Verification items for the finished model (mm, model axes). Face numbers are marked on the shaded views. A direction names the side the tool comes from. Give positions to 0.01 mm unless a question says otherwise; leave off trailing zeros. Write each loop counter-clockwise with the first axis right and the second up, starting at its lowest first coordinate (ties: lowest second). Pieces come first, ordered by that corner, then holes. Notation, with made-up numbers: (-38.75, -38) -> (-23.75, -38) arc R22 cw to (-23.75, 1) -> close; hole circle Ø1 at (55.25, 0). An arc over 180 degrees is marked (long way). Answer as CSV lines item,"result". Start each with the question number.
1) Tool access check on the marked faces 1, 2 and 3. Record the directions out of +Z, -Z, +X, -X, +Y, -Y that give a thin tool (end or side, any length) a straight path to the whole face; none if there is none.
2) Gauge pin test, flat ends, axial feed: pin 1 Ø6 at (y, z) = (17.5, 1) entering from -X; pin 2 Ø6.5 at (x, z) = (41.5, -2) entering from -Y; pin 3 Ø5 at (x, z) = (0, 0) entering from +Y. Record the tip position at first contact, or that the pin passes through.
3) Material ranges on L1, parallel to X at y = 18, z = 0.5; L2, parallel to Z at x = 0, y = 37.1; L3, parallel to X at y = 17, z = 0.5, recorded low to high.
4) Sectioned sample at B-B on x = 16. Record the cut outline in (y, z).
5) Sectioned sample at C-C on x = 0. Record the cut outline in (y, z), and give its area (3 significant figures).
6) Mould release check, pull along Z, two halves, no side actions. Record for the marked faces 4, 5 and 6: released by +Z, released by -Z, zero draft, split by the parting line, or undercut.
7) Sectioned sample at A-A on y = 24.5. Record the cut outline in (x, z), and give its area (3 significant figures).
8) Sectioned sample at D-D on x = 39.5. Record the cut outline in (y, z).
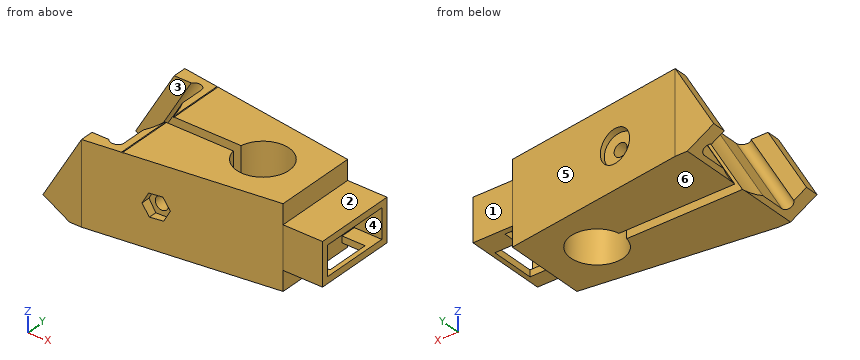
```python
from build123d import *

# Parameters (mm, degrees)
BOSS_EXTRUDE1_DEPTH     = 40
CUT_EXTRUDE1_DEPTH      = 40
SKETCH3_W               = 4.376715803
SKETCH3_H               = 7.921330006
BOSS_EXTRUDE2_DEPTH     = 40
CUT_EXTRUDE2_DEPTH      = 78.145313728
CUT_EXTRUDE2_DEPTH_BACK = 78.145313728
CUT_EXTRUDE3_DEPTH      = 40
CUT_EXTRUDE4_DEPTH      = 43.935998882
CUT_EXTRUDE4_DEPTH_BACK = 43.935998882
SKETCH6_R               = 2
CUT_EXTRUDE5_DEPTH      = 5
SKETCH8_R               = 5
CUT_EXTRUDE6_DEPTH      = 5
CUT_EXTRUDE7_START      = -2
SKETCH9_W               = 6.222682415
SKETCH9_H               = 53.403341902
CUT_EXTRUDE7_DEPTH      = 16
SKETCH10_W              = 13
SKETCH10_H              = 25
SKETCH10_W_2            = 9
SKETCH10_H_2            = 21
BOSS_EXTRUDE3_DEPTH     = 12
CUT_EXTRUDE8_DEPTH      = 11


with BuildPart() as part:
    # Sketch1 → Boss-Extrude1 (new body)
    with BuildSketch(Plane(origin=(0, 0, 0), x_dir=(1, 0, 0), z_dir=(0, 1, 0))):
        Polygon((-35, 12.5), (-20.56624327, -12.5), (35, -12.5), (35, 12.5), align=None)
    extrude(amount=BOSS_EXTRUDE1_DEPTH)

    # Sketch2 → Cut-Extrude1 (cut)
    with BuildSketch(Plane.XY.offset(12.5)):
        Polygon((-20.56624327, 40), (35, 32.5), (35, 40), align=None)
        Polygon((35, 7.5), (-20.56624327, 0), (35, 0), align=None)
    extrude(amount=-CUT_EXTRUDE1_DEPTH, mode=Mode.SUBTRACT)

    # Sketch3 → Boss-Extrude2 (add)
    with BuildSketch(Plane(origin=(-20.837341226, 0, 12.030444566), x_dir=(0.4999999999999981, 0, 0.8660254037844397), z_dir=(-0.8660254037844398, 0, 0.4999999999999982))):
        with Locations((-10.675795445, 21.421253709)):
            Rectangle(SKETCH3_W, SKETCH3_H)
    extrude(amount=BOSS_EXTRUDE2_DEPTH)

    # Sketch4 → Cut-Extrude2 (cut, two sides: drawn at the far end of the back side and taken through both)
    with BuildSketch(Plane(origin=(-4.243718771, 0, -7.350336525), x_dir=(0.8660254037844397, 0, -0.4999999999999983), z_dir=(0.4999999999999982, 0, 0.8660254037844396)).offset(-CUT_EXTRUDE2_DEPTH_BACK)):
        with BuildLine():
            Line((-25.260889132, 35.934120187), (-19.597573928, 35.934120187))
            ThreePointArc((-19.597573928, 35.934120187), (-17.574079433, 36.729704946), (-16.260889132, 34.996783621))
            Line((-16.260889132, 34.996783621), (-16.260889132, 27.623217913))
            ThreePointArc((-16.260889132, 27.623217913), (-14.610889132, 19.996783621), (-16.260889132, 12.37034933))
            Line((-16.260889132, 12.37034933), (-16.260889132, 4.996783621))
            ThreePointArc((-16.260889132, 4.996783621), (-17.574079433, 3.263862297), (-19.597573928, 4.059447055))
            Line((-19.597573928, 4.059447055), (-25.260889132, 4.059447055))
            Line((-25.260889132, 4.059447055), (-25.260889132, 11.549622397))
            Line((-25.260889132, 11.549622397), (-69.354192402, 11.549622397))
            Line((-69.354192402, 11.549622397), (-69.354192402, 27.546843348))
            Line((-69.354192402, 27.546843348), (-25.260889132, 26.613076168))
            Line((-25.260889132, 26.613076168), (-25.260889132, 35.934120187))
        make_face()
    extrude(amount=CUT_EXTRUDE2_DEPTH + CUT_EXTRUDE2_DEPTH_BACK, mode=Mode.SUBTRACT)

    # Sketch5 → Cut-Extrude3 (cut)
    with BuildSketch(Plane(origin=(0, 0, -12.5), x_dir=(-1, 0, 0), z_dir=(0, 0, -1))):
        with BuildLine():
            Line((-11.141275202, 21.5), (29.874932975, 21.5))
            Line((29.874932975, 21.5), (29.874932975, 18.5))
            Line((29.874932975, 18.5), (-11.142492493, 18.5))
            ThreePointArc((-11.142492493, 18.5), (-26.999999341, 20.006434648), (-11.141275202, 21.5))
        make_face()
    extrude(amount=-CUT_EXTRUDE3_DEPTH, mode=Mode.SUBTRACT)

    # Sketch6 → Cut-Extrude4 (cut, two sides: drawn at the far end of the back side and taken through both)
    with BuildSketch(Plane(origin=(0, 18.5, 0), x_dir=(1, 0, 0), z_dir=(0, 1, 0)).offset(-CUT_EXTRUDE4_DEPTH_BACK)):
        Circle(SKETCH6_R)
    extrude(amount=CUT_EXTRUDE4_DEPTH + CUT_EXTRUDE4_DEPTH_BACK, mode=Mode.SUBTRACT)

    # Sketch7 → Cut-Extrude5 (cut)
    with BuildSketch(Plane.XZ):
        Polygon((1.8525736, 3.461402084), (-2.071375338, 3.335076842), (-3.923948938, -0.126325242), (-1.8525736, -3.461402084), (2.071375338, -3.335076842), (3.923948938, 0.126325242), align=None)
    extrude(amount=-CUT_EXTRUDE5_DEPTH, mode=Mode.SUBTRACT)

    # Sketch8 → Cut-Extrude6 (cut)
    with BuildSketch(Plane(origin=(0, 40, 0), x_dir=(1, 0, 0), z_dir=(0, 1, 0))):
        with Locations(Location((0, 0, 0), (0, 0, 270))):
            Circle(SKETCH8_R)
    extrude(amount=-CUT_EXTRUDE6_DEPTH, mode=Mode.SUBTRACT)

    # Sketch9 → Cut-Extrude7 (cut)
    with BuildSketch(Plane(origin=(-14.082343077, 0, 8.130444566), x_dir=(0.4999999999999982, 0, 0.8660254037844397), z_dir=(-0.8660254037844398, 0, 0.4999999999999983)).offset(CUT_EXTRUDE7_START)):
        with Locations((-26.065813196, 19.047949313)):
            Rectangle(SKETCH9_W, SKETCH9_H)
        Polygon((6.045528012, 45.749620264), (6.045528012, -7.653721638), (13.717164193, -7.653721638), (13.717164193, 42.686575292), (13.717164193, 45.749620264), align=None)
    extrude(amount=CUT_EXTRUDE7_DEPTH, mode=Mode.SUBTRACT)

    # Sketch10 → Boss-Extrude3 (add)
    with BuildSketch(Plane(origin=(35, 0, 0), x_dir=(0, 0, -1), z_dir=(1, 0, 0))):
        with Locations((0, 20)):
            Rectangle(SKETCH10_W, SKETCH10_H)
        with Locations((0, 20)):
            Rectangle(SKETCH10_W_2, SKETCH10_H_2, mode=Mode.SUBTRACT)
    extrude(amount=BOSS_EXTRUDE3_DEPTH)

    # Sketch11 → Cut-Extrude8 (cut)
    with BuildSketch(Plane(origin=(0, 0, -6.5), x_dir=(-1, 0, 0), z_dir=(0, 0, -1))):
        Polygon((-38.6, 30.8), (-35, 30.8), (-35, 25.8), (-35, 12.2), (-35, 9.2), (-38.6, 9.2), (-38.6, 12.2), (-45.6, 12.2), (-45.6, 25.8), (-38.6, 25.8), align=None)
    extrude(amount=-CUT_EXTRUDE8_DEPTH, mode=Mode.SUBTRACT)


solid = part.part
```
Ans:
1,face 1,"+Z, -Z, +X, +Y"
1,face 2,"+Z, +X, +Y, -Y"
1,face 3,"+Z, -X"
2,pin 1,"stops at x = -18.31"
2,pin 2,"stops at y = 7.5"
2,pin 3,"stops at y = 35"
3,L1,"x = -16.71 to -1.94, 1.94 to 11.25, 26.75 to 35"
3,L2,"z = -12.5 to -5, 5 to 12.5"
3,L3,"x = -16.87 to -1.94, 1.94 to 11.59, 26.41 to 35"
4,outline,"(4.94, -12.5) -> (12.59, -12.5) -> (12.59, 12.5) -> (4.94, 12.5) -> close; (27.42, -12.5) -> (35.06, -12.5) -> (35.06, 12.5) -> (27.42, 12.5) -> close"
5,outline,"(2.78, -12.5) -> (18.5, -12.5) -> (18.5, -2) -> (5, -2) -> (5, -3.4) -> (2.78, -3.4) -> close; (2.78, 3.4) -> (5, 3.4) -> (5, 2) -> (18.5, 2) -> (18.5, 12.5) -> (2.78, 12.5) -> close; (21.5, -12.5) -> (37.22, -12.5) -> (37.22, -5) -> (35, -5) -> (35, -2) -> (21.5, -2) -> close; (21.5, 2) -> (35, 2) -> (35, 5) -> (37.22, 5) -> (37.22, 12.5) -> (21.5, 12.5) -> close"
5,area,"641 mm²"
6,face 4,"undercut"
6,face 5,"zero draft"
6,face 6,"released by -Z"
7,outline,"(-24.61, -12.29) -> (-24.26, -12.5) -> (12.38, -12.5) -> (12.38, 12.5) -> (-9.25, 12.5) -> (-9.33, 12.37) -> (-9.56, 12.5) -> (-10.3, 12.5) -> close; (25.62, -12.5) -> (35, -12.5) -> (35, 4.5) -> (47, 4.5) -> (47, 6.5) -> (35, 6.5) -> (35, 12.5) -> (25.62, 12.5) -> close; (45.6, -6.5) -> (47, -6.5) -> (47, -4.5) -> (45.6, -4.5) -> close; hole circle Ø4 at (0, 0)"
7,area,"996 mm²"
8,outline,"(7.5, -6.5) -> (12.2, -6.5) -> (12.2, -4.5) -> (9.5, -4.5) -> (9.5, 4.5) -> (30.5, 4.5) -> (30.5, -4.5) -> (25.8, -4.5) -> (25.8, -6.5) -> (32.5, -6.5) -> (32.5, 6.5) -> (7.5, 6.5) -> close"
